from build123d import *

# Parameters (mm, degrees)
SKETCH5_W           = 126
SKETCH5_H           = 22
BOSS_EXTRUDE5_DEPTH = 15
SKETCH6_R           = 1.200912212
CUT_EXTRUDE1_DEPTH  = 10
SKETCH7_R           = 4
CUT_EXTRUDE2_DEPTH  = 16


with BuildPart() as part:
    # Sketch5 → Boss-Extrude5 (new body)
    with BuildSketch(Plane(origin=(0, 0, 0), x_dir=(1, 0, 0), z_dir=(0, 1, 0))):
        with Locations((63, 11)):
            Rectangle(SKETCH5_W, SKETCH5_H)
    extrude(amount=BOSS_EXTRUDE5_DEPTH)

    # Sketch6 → Cut-Extrude1 (cut)
    with BuildSketch(Plane.ZY):
        with Locations((-11.222048747, 2.781464134)):
            Circle(SKETCH6_R)
    extrude(amount=-CUT_EXTRUDE1_DEPTH, mode=Mode.SUBTRACT)

    # Sketch7 → Cut-Extrude2 (cut, through all)
    with BuildSketch(Plane(origin=(0, 15, 0), x_dir=(1, 0, 0), z_dir=(0, 1, 0))):
        with Locations((5, 11)):
            Circle(SKETCH7_R)
        with Locations((121, 11)):
            Circle(SKETCH7_R)
    extrude(amount=-CUT_EXTRUDE2_DEPTH, mode=Mode.SUBTRACT)


solid = part.part
Read the model definition and answer for the solid it produces. Units are mm, in the model's axes. A direction names the side the tool comes from. Give positions to 0.01 mm unless a question says otherwise; leave off trailing zeros. Write each loop counter-clockwise with the first axis right and the second up, starting at its lowest first coordinate (ties: lowest second). Pieces come first, ordered by that corner, then holes. Notation, with made-up numbers: M 49.25,-37 L 107.25,-37 A12 ccw 107.25,-24 Z; hole C 11,-3.5 d9. An arc over 180 degrees is marked long. One line per item, written item: value. Start each with the question number.
(1) Find the intervals of material crossed by line 1 (X direction, y = 7.25, z = -11); line 2 (Z direction, x = 5, y = 10.5); line 3 (X direction, y = 13.25, z = -9.5), in increasing order.
(2) Determine the mould class of faces 3 (the flat face through (62, 15, -11)), 4 (the cylindrical face through (0.48, 2.83, -12.42)), 5 (the flat face through (62, 7, 0)) for opening direction Z: pulls with the +Z half, pulls with the -Z half, needs draft (parallel to the pull), parting line crosses it, or undercut.
(3) Flat-ended cylindrical pins translate along their axes: pin 1 Ø4 at (y, z) = (5, -11) entering from -X; pin 2 Ø0.7 at (y, z) = (3, -11) entering from -X. Find the tip coordinate at first contact, or state that the pin passes through.
(4) A tool of negligible diameter and unlimited length cuts with its end or side. For faces 1 (the flat face through (10, 3, -11)), 2 (the cylindrical face through (118.05, 7.6, -13.7)), from which of +Z, -Z, +X, -X, +Y, -Y can it reach the whole face along a straight path? Write none if from no direction.
(5) Find section A-A (x = 5). Determine the outline of the cut face in (y, z).
Results below:
1. line 1: x = 0 to 1, 9 to 117, 125 to 126
1. line 2: z = -22 to -15, -7 to 0
1. line 3: x = 0 to 1.29, 8.71 to 117.29, 124.71 to 126
2. face 3: needs draft
2. face 4: undercut
2. face 5: pulls with the +Z half
3. pin 1: stops at x = 0
3. pin 2: stops at x = 10
4. face 1: -X
4. face 2: +Y, -Y
5. outline: M 0,-22 L 15,-22 L 15,-15 L 0,-15 Z; M 0,-7 L 15,-7 L 15,0 L 0,0 Z
